```python
from build123d import *

# Parameters (mm, degrees)
ESQUISSE1_R                                 = 30
BOSS_EXTRU_1_DEPTH                          = 10
CHANFREIN1_SIZE                             = 10
CHANFREIN1_SIZE_2                           = 7.002075382
COQUE2_T                                    = -1.5
ESQUISSE2_R                                 = 4
BOSS_EXTRU_2_DEPTH                          = 8.5
CHANFREIN2_SIZE                             = 8.5
CHANFREIN2_SIZE_2                           = 0.445466124
ESQUISSE5_R                                 = 2.554533876
ENL_V_MAT_EXTRU_1_DEPTH                     = 8.5
R_P_TITION_CIRCULAIRE1_COUNT                = 3
CHANFREIN2_OF_R_P_TITION_CIRCULAIRE1_SIZE   = 8.5
CHANFREIN2_OF_R_P_TITION_CIRCULAIRE1_SIZE_2 = 0.445466124


with BuildPart() as part:
    # Esquisse1 → Boss.-Extru.1 (new body)
    with BuildSketch(Plane(origin=(0, 0, 0), x_dir=(1, 0, 0), z_dir=(0, 1, 0))):
        with Locations(Location((0, 0, 0), (0, 0, 270))):
            Circle(ESQUISSE1_R)
    extrude(amount=BOSS_EXTRU_1_DEPTH)

    # Chanfrein1
    # the kernel refuses this chamfer: 10, 7.002075382 mm, written as the material it takes off along each edge
    with BuildSketch(Plane(origin=(0, 10, 0), x_dir=(0, 0, 1), z_dir=(-1, 0, 0))) as chanfrein1_piece_1:
        Polygon((30, -CHANFREIN1_SIZE), (30 - CHANFREIN1_SIZE_2, 0), (30, 0), align=None)
    revolve(axis=Axis((0, 10, 0), (0, 1, 0)), mode=Mode.SUBTRACT)

    # Coque2
    coque2_openings = [part.faces().sort_by_distance(p)[0] for p in [
        (0, 0, 0),
    ]]
    offset(amount=COQUE2_T, openings=coque2_openings, kind=Kind.INTERSECTION)

    # Esquisse2 → Boss.-Extru.2 (add)
    with BuildSketch(Plane.XZ.offset(-8.5)):
        with Locations(Location((-16, 0, 0), (0, 0, 90))):
            Circle(ESQUISSE2_R)
    boss_extru_2 = extrude(amount=BOSS_EXTRU_2_DEPTH)

    # Chanfrein2
    # the kernel refuses this chamfer: 8.5, 0.445466124 mm, written as the material it takes off along each edge
    with BuildSketch(Plane(origin=(-16, 0, 0), x_dir=(0, 0, 1), z_dir=(1, 0, 0))) as chanfrein2_piece_1_section:
        Polygon((4, -CHANFREIN2_SIZE), (4 - CHANFREIN2_SIZE_2, 0), (4, 0), align=None)
    chanfrein2_piece_1 = revolve(axis=Axis((-16, 0, 0), (0, -1, 0)), mode=Mode.PRIVATE)
    chanfrein2_piece_1 = split(chanfrein2_piece_1, bisect_by=Plane(origin=(-16, 8.5, -3.812448858), z_dir=(0, -1, 0)), keep=Keep.TOP, mode=Mode.PRIVATE)
    add(chanfrein2_piece_1, mode=Mode.SUBTRACT)

    # Esquisse5 → Enlèv. mat.-Extru.1 (cut)
    with BuildSketch(Plane.XZ):
        with Locations(Location((-16, 0, 0), (0, 0, 270))):
            Circle(ESQUISSE5_R)
    enl_v_mat_extru_1 = extrude(amount=-ENL_V_MAT_EXTRU_1_DEPTH, mode=Mode.SUBTRACT)

    # Répétition circulaire1: Boss.-Extru.2, Enlèv. mat.-Extru.1 ×3 about axis
    r_p_tition_circulaire1_axis = Axis((0, 0, 0), (0, 1, 0))
    add([boss_extru_2.rotate(r_p_tition_circulaire1_axis, i * 360 / R_P_TITION_CIRCULAIRE1_COUNT) for i in range(1, R_P_TITION_CIRCULAIRE1_COUNT)])
    add([enl_v_mat_extru_1.rotate(r_p_tition_circulaire1_axis, i * 360 / R_P_TITION_CIRCULAIRE1_COUNT) for i in range(1, R_P_TITION_CIRCULAIRE1_COUNT)], mode=Mode.SUBTRACT)

    # Chanfrein2 of Répétition circulaire1
    # the kernel refuses this chamfer: 8.5, 0.445466124 mm, written as the material it takes off along each edge
    with BuildSketch(Plane(origin=(8, 0, 13.856406461), x_dir=(0.8660254037844387, 0, -0.5000000000000001), z_dir=(-0.5000000000000001, 0, -0.8660254037844387))) as chanfrein2_of_r_p_tition_circulaire1_piece_1_section:
        Polygon((4, -CHANFREIN2_OF_R_P_TITION_CIRCULAIRE1_SIZE), (4 - CHANFREIN2_OF_R_P_TITION_CIRCULAIRE1_SIZE_2, 0), (4, 0), align=None)
    chanfrein2_of_r_p_tition_circulaire1_piece_1 = revolve(axis=Axis((8, 0, 13.856406461), (0, -1, 0)), mode=Mode.PRIVATE)
    chanfrein2_of_r_p_tition_circulaire1_piece_1 = split(chanfrein2_of_r_p_tition_circulaire1_piece_1, bisect_by=Plane(origin=(4.698322438, 8.5, 15.762630889), z_dir=(0, -1, 0)), keep=Keep.TOP, mode=Mode.PRIVATE)
    add(chanfrein2_of_r_p_tition_circulaire1_piece_1, mode=Mode.SUBTRACT)
    with BuildSketch(Plane(origin=(8, 0, -13.856406461), x_dir=(-0.8660254037844384, 0, -0.5000000000000003), z_dir=(-0.5000000000000003, 0, 0.8660254037844384))) as chanfrein2_of_r_p_tition_circulaire1_piece_2_section:
        Polygon((4, -CHANFREIN2_OF_R_P_TITION_CIRCULAIRE1_SIZE), (4 - CHANFREIN2_OF_R_P_TITION_CIRCULAIRE1_SIZE_2, 0), (4, 0), align=None)
    chanfrein2_of_r_p_tition_circulaire1_piece_2 = revolve(axis=Axis((8, 0, -13.856406461), (0, -1, 0)), mode=Mode.PRIVATE)
    chanfrein2_of_r_p_tition_circulaire1_piece_2 = split(chanfrein2_of_r_p_tition_circulaire1_piece_2, bisect_by=Plane(origin=(11.301677562, 8.5, -11.950182032), z_dir=(0, -1, 0)), keep=Keep.TOP, mode=Mode.PRIVATE)
    add(chanfrein2_of_r_p_tition_circulaire1_piece_2, mode=Mode.SUBTRACT)


solid = part.part
```
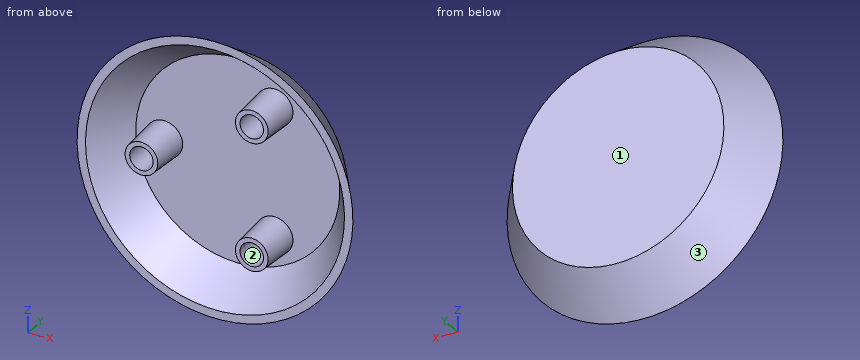
Could you check a few things on this model? Use its own coordinates, in mm. Face numbers are marked on the shaded views. Round coordinates to 2 decimals unless told otherwise and drop trailing zeros. Loops run counter-clockwise (first coordinate to the right, second up) from the corner with the lowest first, then second, coordinate; pieces in that order, holes last.
Q1. Please list where these lines run through material, in increasing order: L1, parallel to X at y = 6.75, z = -16; L2, parallel to X at y = 3, z = -12; L3, parallel to Z at x = 8.5, y = 8.25.
Q2. Thinking about a two-plate mould opening in X: for the marked faces 1, 2 and 3, which applies, pulls with the +X half, pulls with the -X half, needs draft (parallel to the pull), parting line crosses it, or undercut?
Q3. I want a section at B-B (z = 0). Write out the boundary of the cut face in (x, y), and give its area (3 significant figures).
Q4. I want a section at A-A (y = 3.75). Write out the boundary of the cut face in (x, z).
Q5. For P1, Ø6, axis at x = 16.5, z = -15.5, coming from the -Y side; P2, Ø1.5, axis at x = 8, z = -14, coming from the -Y side; P3, Ø1, axis at y = 2.5, z = -19, coming from the +X side, each with a flat end and sliding along its axis, tell me the tip position at first contact or that it passes through.
Answer below:
1. L1: x = -19.56 to -17.13, 4.73 to 6.61, 9.39 to 11.27, 17.13 to 19.56
1. L2: x = -25.19 to -23.14, 4.79 to 6.25, 9.75 to 11.21, 23.14 to 25.19
1. L3: z = -22.68 to -20.72, -17.81 to -16.36, -11.35 to -9.9, 9.9 to 11.35, 16.36 to 17.81, 20.72 to 22.68
2. face 1: needs draft
2. face 2: undercut
2. face 3: parting line crosses it
3. outline: (-30, 0) - (-28.17, 0) - (-22.22, 8.5) - (-20, 8.5) - (-19.55, 0) - (-18.55, 0) - (-18.55, 8.5) - (-13.45, 8.5) - (-13.45, 0) - (-12.45, 0) - (-12, 8.5) - (22.22, 8.5) - (28.17, 0) - (30, 0) - (23, 10) - (-23, 10) - close
3. area: 122 mm2
4. outline: circle Ø54.75 at (0, 0); circle Ø7.5 at (-16, 0); circle Ø7.5 at (8, -13.86); circle Ø7.5 at (8, 13.86); hole circle Ø51.09 at (0, 0); hole circle Ø5.11 at (-16, 0); hole circle Ø5.11 at (8, -13.86); hole circle Ø5.11 at (8, 13.86)
5. P1: stops at y = 3.61
5. P2: stops at y = 8.5
5. P3: stops at x = 21.55
